Could you check a few things on this model? Use its own coordinates, in mm. A direction names the side the tool comes from. Round coordinates to 2 decimals unless told otherwise and drop trailing zeros. Order: outer loops, then holes, each group sorted by start corner. A loop starts at its lowest first (then second) coordinate and runs counter-clockwise, first axis right, second up.
```python
from build123d import *

# Parameters (mm, degrees)
F1_DEPTH = 25
F2_R     = 4
F3_DEPTH = 12.5


with BuildPart() as f1:
    # F0 (on Front) → F1 (new body)
    with BuildSketch(Plane.XZ):
        with BuildLine():
            Line((-12.5, 12.5), (-65, 12.5))
            Line((-65, 12.5), (-65, 4.999099))
            Line((-65, 4.999099), (-25.094896, 4.999099))
            ThreePointArc((-25.094896, 4.999099), (-20.000005, 0.006726), (-25.081447, -4.999337))
            Line((-25.081447, -4.999337), (-65, -4.999337))
            Line((-65, -4.999337), (-65, -12.5))
            Line((-65, -12.5), (-12.5, -12.5))
            Line((-12.5, -12.5), (-12.5, -10))
            Line((-12.5, -10), (12.5, -10))
            Line((12.5, -10), (12.5, -12.5))
            Line((12.5, -12.5), (65, -12.5))
            Line((65, -12.5), (65, -4.999337))
            Line((65, -4.999337), (25.081447, -4.999337))
            ThreePointArc((25.081447, -4.999337), (20.000005, 0.006726), (25.094896, 4.999099))
            Line((25.094896, 4.999099), (65, 4.999099))
            Line((65, 4.999099), (65, 12.5))
            Line((65, 12.5), (12.5, 12.5))
            Line((12.5, 12.5), (12.5, 10))
            Line((12.5, 10), (0, 10))
            Line((0, 10), (-12.5, 10))
            Line((-12.5, 10), (-12.5, 12.5))
        make_face()
        with BuildLine():
            ThreePointArc((6, 0), (-4.242641, -4.242641), (0, 6))
            ThreePointArc((0, 6), (4.242641, 4.242641), (6, 0))
        make_face(mode=Mode.SUBTRACT)
    extrude(amount=F1_DEPTH)

    # F2 (on Top) → F3 (cut, symmetric)
    with BuildSketch(Plane.XY):
        with Locations((-50, -12.5)):
            Circle(F2_R)
        with Locations((50, -12.5)):
            Circle(F2_R)
    extrude(amount=F3_DEPTH, both=True, mode=Mode.SUBTRACT)


solid = f1.part
```
Q1. I need wall thicknesses on L1, parallel to Y at x = 50, z = -7.5; L2, parallel to Z at x = 0, y = -11; L3, parallel to Z at x = 47.5, y = -5.75. Which ranges of each line are inside material? Lowest first, please.
Q2. Imagine slicing it at C-C, the plane z = 8. Please give me the cut outline in (x, y).
Q3. Imagine slicing it at B-B, the plane y = -5.25. Please give me the cut outline in (x, z), then the cut area to 3 significant figures.
Q4. We'd pull the mould along Z, two halves only. Please class faces 1 (the cylindrical face through (-53.996, -12.324, -8.697)), 2 (the flat face through (-45, -12, 4.999)), 3 (the flat face through (39, -12, 12.5)), 4 (the flat face through (45, -12, 4.999)): released by +Z, released by -Z, zero draft, split by the parting line, or undercut.
Q5. For P1, Ø12, axis at x = -51, z = -1, coming from the -Y side; P2, Ø1.5, axis at y = -18.5, z = 2, coming from the +X side, each with a flat end and sliding along its axis, tell me the tip position at first contact or that it passes through.
Q6. Imagine slicing it at A-A, the plane x = -55.5. Please give me the cut outline in (y, z).
Q7. Imagine slicing it at D-D, the plane x = 50. Please give me the cut outline in (y, z), then the cut area to 3 significant figures.
Q8. For faces 5 (the flat face through (0, -12, 10)), 6 (the flat face through (-45, -12, -4.999)), 7 (the cylindrical face through (46.004, -12.324, -8.697)), 8 (the flat face through (45, -12, -4.999)), 9 (the flat face through (-12.5, -12, -11)), which set-ups out of +Z, -Z, +X, -X, +Y, -Y let a thin tool reach every point of the face, with its end or its side?
Filled in:
1. L1: y = -25 to -16.5, -8.5 to 0
1. L2: z = -10 to -6, 6 to 10
1. L3: z = -12.5 to -5, 5 to 12.5
2. outline: (-65, -25) - (65, -25) - (65, 0) - (-65, 0) - close; hole circle Ø8 at (-50, -12.5); hole circle Ø8 at (50, -12.5)
3. outline: (-65, -12.5) - (-12.5, -12.5) - (-12.5, -10) - (12.5, -10) - (12.5, -12.5) - (65, -12.5) - (65, -5) - (25.08, -5) arc R5 cw (long way) to (25.09, 5) - (65, 5) - (65, 12.5) - (12.5, 12.5) - (12.5, 10) - (-12.5, 10) - (-12.5, 12.5) - (-65, 12.5) - (-65, 5) - (-25.09, 5) arc R5 cw (long way) to (-25.08, -5) - (-65, -5) - close; hole (0, 6) arc R6 ccw (long way) to (6, 0) arc R6 ccw to start
3. area: 2,130 mm2
4. face 1: zero draft
4. face 2: undercut
4. face 3: released by +Z
4. face 4: undercut
5. P1: stops at y = -25
5. P2: stops at x = 20.82
6. outline: (-25, -12.5) - (0, -12.5) - (0, -5) - (-25, -5) - close; (-25, 5) - (0, 5) - (0, 12.5) - (-25, 12.5) - close
7. outline: (-25, -12.5) - (-16.5, -12.5) - (-16.5, -5) - (-25, -5) - close; (-25, 5) - (-16.5, 5) - (-16.5, 12.5) - (-25, 12.5) - close; (-8.5, -12.5) - (0, -12.5) - (0, -5) - (-8.5, -5) - close; (-8.5, 5) - (0, 5) - (0, 12.5) - (-8.5, 12.5) - close
7. area: 255 mm2
8. face 5: +Z, +Y, -Y
8. face 6: -X, +Y, -Y
8. face 7: +Z, -Z
8. face 8: +X, +Y, -Y
8. face 9: -Z, +Y, -Y
